```python
from build123d import *

# Parameters (mm, degrees)
BOSS_EXTRUDE1_DEPTH = 38.1
FILLET1_R           = 0.508
FILLET2_R           = 0.127
CHAMFER1_SIZE       = 0.3
FILLET3_R           = 0.127


with BuildPart() as part:
    # Sketch1 → Boss-Extrude1 (new body)
    with BuildSketch(Plane.XY):
        Polygon((0, 0), (5.715, 0), (5.715, 38.1), (0, 38.1), (0, 20.828), (-6.604, 20.828), (-6.604, 22.4155), (-8.1915, 20.828), (-8.1915, 19.2405), (0, 19.2405), (0, 14.097), (-8.1915, 14.097), (-8.1915, 10.922), (0, 10.922), align=None)
    extrude(amount=BOSS_EXTRUDE1_DEPTH)

    # Fillet1
    fillet1_edges = [part.edges().sort_by_distance(p)[0] for p in [
        (0, 0, 19.05),
        (0, 10.922, 19.05),
        (-8.1915, 10.922, 19.05),
        (-8.1915, 14.097, 19.05),
        (0, 14.097, 19.05),
        (0, 19.2405, 19.05),
        (-8.1915, 19.2405, 19.05),
        (-8.1915, 20.828, 19.05),
        (-6.604, 20.828, 19.05),
        (0, 20.828, 19.05),
        (0, 38.1, 19.05),
        (5.715, 38.1, 19.05),
        (5.715, 0, 19.05),
    ]]
    fillet(fillet1_edges, radius=FILLET1_R)

    # Fillet2
    fillet2_edges = [part.edges().sort_by_distance(p)[0] for p in [
        (-6.604, 22.4155, 19.05),
    ]]
    fillet(fillet2_edges, radius=FILLET2_R)

    # Chamfer1
    # the kernel refuses this chamfer: 0.3 mm, written as the material it takes off along each edge
    with BuildSketch(Plane(origin=(-6.275266217, 22.744233783, 0), x_dir=(0.7068394360706772, -0.7068394360706697, -0.02749587661058634), z_dir=(-0.7071067811865438, -0.7071067811865513, 0))) as chamfer1_piece_1:
        Polygon((CHAMFER1_SIZE * 0.999621916911, CHAMFER1_SIZE * 0.0274958766106), (-CHAMFER1_SIZE * 0.0274958766106, CHAMFER1_SIZE * 0.999621916911), (0, 0), align=None)
    extrude(amount=2.499543315, mode=Mode.SUBTRACT)
    with BuildSketch(Plane(origin=(-7.6835, 19.2405, 0), x_dir=(0, 0.9996219169112968, -0.02749587661058633), z_dir=(1, 0, 0)), Plane(origin=(-7.6835, 10.922, 0), x_dir=(0, 0.9996219169112968, -0.02749587661058633), z_dir=(1, 0, 0)), Plane(origin=(-0.508, 14.097, 0), x_dir=(0, -0.9996219169112968, -0.02749587661058633), z_dir=(-1, 0, 0))) as chamfer1_piece_2:
        Polygon((CHAMFER1_SIZE * 0.999621916911, CHAMFER1_SIZE * 0.0274958766106), (-CHAMFER1_SIZE * 0.0274958766106, CHAMFER1_SIZE * 0.999621916911), (0, 0), align=None)
    extrude(amount=7.1755, mode=Mode.SUBTRACT)
    with BuildSketch(Plane(origin=(0.508, 0, 0), x_dir=(0, 0.9996219169112968, -0.027495876610586275), z_dir=(1, 0, 0)), Plane(origin=(5.207, 38.1, 0), x_dir=(0, -0.9996219169112968, -0.027495876610586494), z_dir=(-1, 0, 0))) as chamfer1_piece_3:
        Polygon((CHAMFER1_SIZE * 0.999621916911, CHAMFER1_SIZE * 0.0274958766106), (-CHAMFER1_SIZE * 0.0274958766106, CHAMFER1_SIZE * 0.999621916911), (0, 0), align=None)
    extrude(amount=4.699, mode=Mode.SUBTRACT)
    with BuildSketch(Plane(origin=(0, 10.414, 0), x_dir=(0.9996219169112968, 0, -0.02749587661058637), z_dir=(0, -1, 0))) as chamfer1_piece_4:
        Polygon((CHAMFER1_SIZE * 0.999621916911, CHAMFER1_SIZE * 0.0274958766106), (-CHAMFER1_SIZE * 0.0274958766106, CHAMFER1_SIZE * 0.999621916911), (0, 0), align=None)
    extrude(amount=9.906, mode=Mode.SUBTRACT)
    with BuildSketch(Plane(origin=(-8.1915, 13.589, 0), x_dir=(0.9996219169112968, 0, -0.02749587661058637), z_dir=(0, -1, 0))) as chamfer1_piece_5:
        Polygon((CHAMFER1_SIZE * 0.999621916911, CHAMFER1_SIZE * 0.0274958766106), (-CHAMFER1_SIZE * 0.0274958766106, CHAMFER1_SIZE * 0.999621916911), (0, 0), align=None)
    extrude(amount=2.159, mode=Mode.SUBTRACT)
    with BuildSketch(Plane(origin=(0, 18.7325, 0), x_dir=(0.9996219169112968, 0, -0.02749587661058637), z_dir=(0, -1, 0))) as chamfer1_piece_6:
        Polygon((CHAMFER1_SIZE * 0.999621916911, CHAMFER1_SIZE * 0.0274958766106), (-CHAMFER1_SIZE * 0.0274958766106, CHAMFER1_SIZE * 0.999621916911), (0, 0), align=None)
    extrude(amount=4.1275, mode=Mode.SUBTRACT)
    with BuildSketch(Plane(origin=(-8.1915, 20.61757951, 0), x_dir=(0.9996219169112968, 1.118541876484896e-15, -0.02749587661058637), z_dir=(0, -1, 0))) as chamfer1_piece_7:
        Polygon((CHAMFER1_SIZE * 0.999621916911, CHAMFER1_SIZE * 0.0274958766106), (-CHAMFER1_SIZE * 0.0274958766106, CHAMFER1_SIZE * 0.999621916911), (0, 0), align=None)
    extrude(amount=0.86907951, mode=Mode.SUBTRACT)
    with BuildSketch(Plane(origin=(-6.604, 21.336, 0), x_dir=(-0.9996219169112968, 0, -0.02749587661058637), z_dir=(0, 1, 0))) as chamfer1_piece_8:
        Polygon((CHAMFER1_SIZE * 0.999621916911, CHAMFER1_SIZE * 0.0274958766106), (-CHAMFER1_SIZE * 0.0274958766106, CHAMFER1_SIZE * 0.999621916911), (0, 0), align=None)
    extrude(amount=1.544399774, mode=Mode.SUBTRACT)
    with BuildSketch(Plane(origin=(-0.508, 20.828, 0), x_dir=(0, -0.9996219169112968, -0.02749587661058633), z_dir=(-1, 0, 0))) as chamfer1_piece_9:
        Polygon((CHAMFER1_SIZE * 0.999621916911, CHAMFER1_SIZE * 0.0274958766106), (-CHAMFER1_SIZE * 0.0274958766106, CHAMFER1_SIZE * 0.999621916911), (0, 0), align=None)
    extrude(amount=5.588, mode=Mode.SUBTRACT)
    with BuildSketch(Plane(origin=(0, 37.592, 0), x_dir=(0.9996219169112968, 0, -0.02749587661058637), z_dir=(0, -1, 0))) as chamfer1_piece_10:
        Polygon((CHAMFER1_SIZE * 0.999621916911, CHAMFER1_SIZE * 0.0274958766106), (-CHAMFER1_SIZE * 0.0274958766106, CHAMFER1_SIZE * 0.999621916911), (0, 0), align=None)
    extrude(amount=16.256, mode=Mode.SUBTRACT)
    with BuildSketch(Plane(origin=(5.715, 0.508, 0), x_dir=(-0.9996219169112968, 0, -0.02749587661058637), z_dir=(0, 1, 0))) as chamfer1_piece_11:
        Polygon((CHAMFER1_SIZE * 0.999621916911, CHAMFER1_SIZE * 0.0274958766106), (-CHAMFER1_SIZE * 0.0274958766106, CHAMFER1_SIZE * 0.999621916911), (0, 0), align=None)
    extrude(amount=37.084, mode=Mode.SUBTRACT)
    with BuildSketch(Plane(origin=(-7.6835, 13.589, 0), x_dir=(0, 1, 0), z_dir=(1, 0, 0))) as chamfer1_piece_12:
        Polygon((0.508 - CHAMFER1_SIZE, 0), (0.508, CHAMFER1_SIZE), (0.508, 0), align=None)
    revolve(axis=Axis((-7.6835, 13.589, 0), (0, 0, 1)), revolution_arc=90, mode=Mode.SUBTRACT)
    with BuildSketch(Plane(origin=(-7.6835, 11.43, 0), x_dir=(-1, 0, 0), z_dir=(0, 1, 0))) as chamfer1_piece_13:
        Polygon((0.508 - CHAMFER1_SIZE, 0), (0.508, CHAMFER1_SIZE), (0.508, 0), align=None)
    revolve(axis=Axis((-7.6835, 11.43, 0), (0, 0, 1)), revolution_arc=90, mode=Mode.SUBTRACT)
    with BuildSketch(Plane(origin=(0.508, 0.508, 0), x_dir=(0, -1, 0), z_dir=(1, 0, 0))) as chamfer1_piece_14:
        Polygon((0.508 - CHAMFER1_SIZE, 0), (0.508, -CHAMFER1_SIZE), (0.508, 0), align=None)
    revolve(axis=Axis((0.508, 0.508, 0), (0, 0, -1)), revolution_arc=90, mode=Mode.SUBTRACT)
    with BuildSketch(Plane(origin=(0.508, 37.592, 0), x_dir=(0, 1, 0), z_dir=(1, 0, 0))) as chamfer1_piece_15:
        Polygon((0.508 - CHAMFER1_SIZE, 0), (0.508, CHAMFER1_SIZE), (0.508, 0), align=None)
    revolve(axis=Axis((0.508, 37.592, 0), (0, 0, 1)), revolution_arc=90, mode=Mode.SUBTRACT)
    with BuildSketch(Plane(origin=(5.207, 0.508, 0), x_dir=(0, -1, 0), z_dir=(-1, 0, 0))) as chamfer1_piece_16:
        Polygon((0.508 - CHAMFER1_SIZE, 0), (0.508, CHAMFER1_SIZE), (0.508, 0), align=None)
    revolve(axis=Axis((5.207, 0.508, 0), (0, 0, 1)), revolution_arc=90, mode=Mode.SUBTRACT)
    with BuildSketch(Plane(origin=(5.207, 37.592, 0), x_dir=(1, 0, 0), z_dir=(0, -1, 0))) as chamfer1_piece_17:
        Polygon((0.508 - CHAMFER1_SIZE, 0), (0.508, CHAMFER1_SIZE), (0.508, 0), align=None)
    revolve(axis=Axis((5.207, 37.592, 0), (0, 0, 1)), revolution_arc=90, mode=Mode.SUBTRACT)
    with BuildSketch(Plane(origin=(-7.6835, 20.61757951, 0), x_dir=(-0.7071067811865519, 0.7071067811865432, 0), z_dir=(0.7071067811865432, 0.7071067811865519, 0))) as chamfer1_piece_18:
        Polygon((0.508 - CHAMFER1_SIZE, 0), (0.508, CHAMFER1_SIZE), (0.508, 0), align=None)
    revolve(axis=Axis((-7.6835, 20.61757951, 0), (0, 0, 1)), revolution_arc=45, mode=Mode.SUBTRACT)
    with BuildSketch(Plane(origin=(-7.6835, 19.7485, 0), x_dir=(-1, 0, 0), z_dir=(0, 1, 0))) as chamfer1_piece_19:
        Polygon((0.508 - CHAMFER1_SIZE, 0), (0.508, CHAMFER1_SIZE), (0.508, 0), align=None)
    revolve(axis=Axis((-7.6835, 19.7485, 0), (0, 0, 1)), revolution_arc=90, mode=Mode.SUBTRACT)
    with BuildSketch(Plane(origin=(-0.508, 14.605, 0), x_dir=(1, 0, 0), z_dir=(0, 1, 0))) as chamfer1_piece_20:
        Polygon((0.508 + CHAMFER1_SIZE, 0), (0.508, -CHAMFER1_SIZE), (0.508, 0), align=None)
    revolve(axis=Axis((-0.508, 14.605, 0), (0, 0, -1)), revolution_arc=90, mode=Mode.SUBTRACT)
    with BuildSketch(Plane(origin=(-0.508, 18.7325, 0), x_dir=(0, 1, 0), z_dir=(-1, 0, 0))) as chamfer1_piece_21:
        Polygon((0.508 + CHAMFER1_SIZE, 0), (0.508, -CHAMFER1_SIZE), (0.508, 0), align=None)
    revolve(axis=Axis((-0.508, 18.7325, 0), (0, 0, -1)), revolution_arc=90, mode=Mode.SUBTRACT)
    with BuildSketch(Plane(origin=(-0.508, 10.414, 0), x_dir=(0, 1, 0), z_dir=(-1, 0, 0))) as chamfer1_piece_22:
        Polygon((0.508 + CHAMFER1_SIZE, 0), (0.508, -CHAMFER1_SIZE), (0.508, 0), align=None)
    revolve(axis=Axis((-0.508, 10.414, 0), (0, 0, -1)), revolution_arc=90, mode=Mode.SUBTRACT)
    with BuildSketch(Plane(origin=(-6.096, 21.336, 0), x_dir=(0, -1, 0), z_dir=(1, 0, 0))) as chamfer1_piece_23:
        Polygon((0.508 + CHAMFER1_SIZE, 0), (0.508, -CHAMFER1_SIZE), (0.508, 0), align=None)
    revolve(axis=Axis((-6.096, 21.336, 0), (0, 0, -1)), revolution_arc=90, mode=Mode.SUBTRACT)
    with BuildSketch(Plane(origin=(-0.508, 21.336, 0), x_dir=(1, 0, 0), z_dir=(0, 1, 0))) as chamfer1_piece_24:
        Polygon((0.508 + CHAMFER1_SIZE, 0), (0.508, -CHAMFER1_SIZE), (0.508, 0), align=None)
    revolve(axis=Axis((-0.508, 21.336, 0), (0, 0, -1)), revolution_arc=90, mode=Mode.SUBTRACT)

    # Fillet3
    fillet3_edges = [part.edges().sort_by_distance(p)[0] for p in [
        (-7.431756403, 21.587743597, 38.1),
        (-6.682399204, 22.226227578, 38.1),
        (-4.09575, 19.2405, 38.1),
        (-8.1915, 20.183039755, 38.1),
        (2.8575, 0, 38.1),
        (5.715, 19.05, 38.1),
        (2.8575, 38.1, 38.1),
        (0, 29.464, 38.1),
        (-3.302, 20.828, 38.1),
        (-6.604, 21.722447439, 38.1),
        (0, 16.66875, 38.1),
        (-4.09575, 14.097, 38.1),
        (-8.1915, 12.5095, 38.1),
        (-4.09575, 10.922, 38.1),
        (0, 5.461, 38.1),
        (-8.042710245, 13.948210245, 38.1),
        (-8.042710245, 11.070789755, 38.1),
        (0.148789755, 0.148789755, 38.1),
        (0.148789755, 37.951210245, 38.1),
        (5.566210245, 0.148789755, 38.1),
        (5.566210245, 37.951210245, 38.1),
        (-8.152830803, 20.811982694, 38.1),
        (-8.042710245, 19.389289755, 38.1),
        (-0.148789755, 14.245789755, 38.1),
        (-0.148789755, 19.091710245, 38.1),
        (-0.148789755, 10.773210245, 38.1),
        (-6.455210245, 20.976789755, 38.1),
        (-0.148789755, 20.976789755, 38.1),
    ]]
    fillet(fillet3_edges, radius=FILLET3_R)


solid = part.part
```
Verification items for the finished model (mm, model axes). A direction names the side the tool comes from. Coordinates: 2 decimals unless noted, no trailing zeros. Write each loop counter-clockwise with the first axis right and the second up, starting at its lowest first coordinate (ties: lowest second). Pieces come first, ordered by that corner, then holes. Notation, with made-up numbers: M 40.5,-9.5 L 96.5,-9.5 A24 ccw 96.5,23.5 Z; hole C 15,79 d7. An arc over 180 degrees is marked long. Answer as a JSON object with one key per item and string values. Group by question number.
(1) Cross-section at A-A, the plane x = -3.5. Record the cut outline in (y, z).
(2) Cross-section at B-B, the plane y = 5. Record the cut outline in (x, z) (3 decimals).
(3) Gauge pin test, flat ends, axial feed: pin 1 (2 mm diameter, centred on x = -2, z = 7, fed in from -Y); pin 2 (1.2 mm diameter, centred on y = 17.5, z = 10.5, fed in from -X); pin 3 (4 mm diameter, centred on x = -4.5, y = 15, fed in from -Z); pin 4 (5.5 mm diameter, centred on x = -2.5, z = 9.5, fed in from -Y). Record the tip position at first contact, or that the pin passes through.
(4) Release check for a two-part mould opening along Y. For faces 4 (the face through (-4, 10.922, 19)), 5 (the face through (0, 6, 19)), 6 (the face through (-4, 19.24, 19)) record: +Y half, -Y half, draft (parallel to the pull), parting line (faces both ways), or undercut.
(5) Material ranges on line 1 (Y direction, x = -0.5, z = 27.5); line 2 (X direction, y = 5.5, z = 32) (3 decimals); line 3 (Y direction, x = -6.75, z = 18.5), recorded low to high.
(6) Tool access check on faces 1 (the face through (3, 0, 19)), 2 (the face through (-4, 14.097, 19)), 3 (the face through (-3, 20.828, 19)). Record the directions out of +Z, -Z, +X, -X, +Y, -Y that give a thin tool (end or side, any length) a straight path to the whole face; none if there is none.
Reply:
{
 "1": {"outline": "M 10.92,0.3 L 11.22,0 L 13.8,0 L 14.1,0.3 L 14.1,37.97 A0.13 ccw 13.97,38.1 L 11.05,38.1 A0.13 ccw 10.92,37.97 Z; M 19.24,0.3 L 19.54,0 L 20.53,0 L 20.83,0.3 L 20.83,37.97 A0.13 ccw 20.7,38.1 L 19.37,38.1 A0.13 ccw 19.24,37.97 Z"},
 "2": {"outline": "M 0,0.3 L 0.3,0 L 5.415,0 L 5.715,0.3 L 5.715,37.973 A0.127 ccw 5.588,38.1 L 0.127,38.1 A0.127 ccw 0,37.973 Z"},
 "3": {"pin 1": "y = 10.92", "pin 2": "x = 0", "pin 3": "z = 0", "pin 4": "y = 0.07"},
 "4": {"face 4": "-Y half", "face 5": "draft", "face 6": "undercut"},
 "5": {"line 1": "10.92 to 14.1, 19.24 to 20.83", "line 2": "0 to 5.715", "line 3": "10.92 to 14.1, 19.24 to 22.23"},
 "6": {"face 1": "+Z, -Z, +X, -X, -Y", "face 2": "+Z, -Z, -X", "face 3": "+Z, -Z, +Y"}
}
